Read the model definition and answer for the solid it produces. Units are mm, in the model's axes. Face numbers are marked on the shaded views. A direction names the side the tool comes from. Give positions to 0.01 mm unless a question says otherwise; leave off trailing zeros. Loops run counter-clockwise (first coordinate to the right, second up) from the corner with the lowest first, then second, coordinate; pieces in that order, holes last. Notation, with made-up numbers: (-34.5, 21) -> (-28.5, 21) arc R30 ccw to (-28.5, 52) -> close; hole circle Ø6 at (48.5, 76). An arc over 180 degrees is marked (long way). One line per item, written item: value. Start each with the question number.
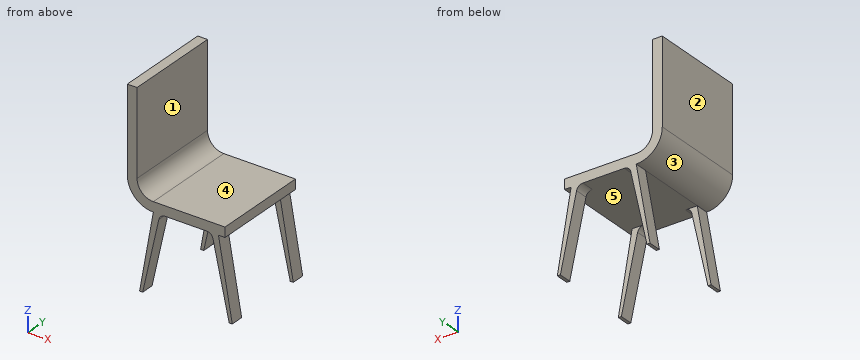
from build123d import *

# Parameters (mm, degrees)
F1_DEPTH = 190.5
F3_DEPTH = 50.8


with BuildPart() as f1:
    # F0 (on Front) → F1 (new body, symmetric)
    with BuildSketch(Plane.XZ):
        with BuildLine():
            Line((-342.9, 431.8), (-381, 431.8))
            Line((-381, 431.8), (-381, 101.6))
            ThreePointArc((-381, 101.6), (-351.2420489686, 29.7579510314), (-279.4, 0))
            Line((-279.4, 0), (0, 0))
            Line((0, 0), (0, 38.1))
            Line((0, 38.1), (-279.4, 38.1))
            ThreePointArc((-279.4, 38.1), (-324.3012806053, 56.6987193947), (-342.9, 101.6))
            Line((-342.9, 101.6), (-342.9, 431.8))
        make_face()
    extrude(amount=F1_DEPTH, both=True)

    # F2 (on face) → F3 (join)
    with BuildSketch(Plane.XZ.offset(190.5)):
        with BuildLine():
            Line((-279.4, 0), (-333.1444637199, -304.8))
            Line((-333.1444637199, -304.8), (-321.1806972317, -304.8))
            Line((-321.1806972317, -304.8), (-258.0204274065, -19.902433806))
            ThreePointArc((-258.0204274065, -19.902433806), (-249.1209650191, -5.5909341294), (-233.2225088256, 0))
            Line((-233.2225088256, 0), (-279.4, 0))
        make_face()
        with BuildLine():
            Line((-25.4, 0), (-71.5774911744, 0))
            ThreePointArc((-71.5774911744, 0), (-55.6790349809, -5.5909341294), (-46.7795725935, -19.902433806))
            Line((-46.7795725935, -19.902433806), (16.3806972317, -304.8))
            Line((16.3806972317, -304.8), (28.3444637199, -304.8))
            Line((28.3444637199, -304.8), (-25.4, 0))
        make_face()
    extrude(amount=-F3_DEPTH)

    # F4: F1 across plane


with BuildPart() as f1_1:
    add(f1.part)
    add(f1.part.mirror(Plane.XZ))


solid = f1_1.part
Item 1: Section A-A, the plane x = -293.5 is taken. Determine the outline of the cut face in (y, z).
Item 2: For the marked faces 1 and 2, determine the directions among +Z, -Z, +X, -X, +Y, -Y from which every point of the face is accessible in a straight line to the end or side of a thin tool.
Item 3: Flat-ended cylindrical pins translate along their axes: pin 1 (12 mm diameter, centred on x = -136, y = -137.5, fed in from -Z); pin 2 (10 mm diameter, centred on y = -26.5, z = 26, fed in from +X); pin 3 (1 mm diameter, centred on y = 30, z = 236, fed in from +X). Find the tip coordinate at first contact, or state that the pin passes through.
Item 4: Section D-D, the plane z = -55.5 is taken. Determine the outline of the cut face in (x, y).
Item 5: Determine the mould class of the marked faces 3, 4 and 5 for opening direction X: pulls with the +X half, pulls with the -X half, needs draft (parallel to the pull), parting line crosses it, or undercut.
Item 6: Section C-C, the plane y = -18 is taken. Determine the outline of the cut face in (x, z), plus the area to 3 significant figures.
Item 7: Consider L1, parallel to Y at x = -293, z = -132; L2, parallel to X at y = 66, z = 371.5; L3, parallel to Z at x = -77, y = -8. Determine where each line is inside the solid, lowest interval first. Write a range as [from, to].
Item 8: Section B-B, the plane z = -149.5 is taken. Determine the outline of the cut face in (x, y), plus the area to 3 significant figures.
Computed values:
1. outline: (-190.5, -179.94) -> (-139.7, -179.94) -> (-139.7, -79.97) -> (-190.5, -79.97) -> close; (-190.5, 0.98) -> (190.5, 0.98) -> (190.5, 39.69) -> (-190.5, 39.69) -> close; (139.7, -179.94) -> (190.5, -179.94) -> (190.5, -79.97) -> (139.7, -79.97) -> close
2. face 1: +Z, +X, +Y, -Y
2. face 2: +Z, -Z, -X, +Y, -Y
3. pin 1: z = 0
3. pin 2: x = 0
3. pin 3: x = -342.9
4. outline: (-289.19, -190.5) -> (-265.91, -190.5) -> (-265.91, -139.7) -> (-289.19, -139.7) -> close; (-289.19, 139.7) -> (-265.91, 139.7) -> (-265.91, 190.5) -> (-289.19, 190.5) -> close; (-38.89, -190.5) -> (-15.61, -190.5) -> (-15.61, -139.7) -> (-38.89, -139.7) -> close; (-38.89, 139.7) -> (-15.61, 139.7) -> (-15.61, 190.5) -> (-38.89, 190.5) -> close
5. face 3: pulls with the -X half
5. face 4: needs draft
5. face 5: undercut
6. outline: (-381, 101.6) arc R101.6 ccw to (-279.4, 0) -> (0, 0) -> (0, 38.1) -> (-279.4, 38.1) arc R63.5 cw to (-342.9, 101.6) -> (-342.9, 431.8) -> (-381, 431.8) -> close
6. area: 28,200 mm²
7. L1: [-190.5, -139.7], [139.7, 190.5]
7. L2: [-381, -342.9]
7. L3: [0, 38.1]
8. outline: (-305.76, -190.5) -> (-286.75, -190.5) -> (-286.75, -139.7) -> (-305.76, -139.7) -> close; (-305.76, 139.7) -> (-286.75, 139.7) -> (-286.75, 190.5) -> (-305.76, 190.5) -> close; (-18.05, -190.5) -> (0.96, -190.5) -> (0.96, -139.7) -> (-18.05, -139.7) -> close; (-18.05, 139.7) -> (0.96, 139.7) -> (0.96, 190.5) -> (-18.05, 190.5) -> close
8. area: 3,860 mm²
